from build123d import *

# Parameters (mm, degrees)
F0_W      = 125
F0_H      = 110
F1_DEPTH  = 200
F2_W      = 115.000002
F2_H      = 190.000002
F3_DEPTH  = 95
F4_R      = 2
F5_R      = 20
F7_DEPTH  = 200.001
F6_R      = 12.5
F8_DEPTH  = 200.001
F9_W      = 3
F9_H      = 190.000002
F10_DEPTH = 95


with BuildPart() as f1:
    # F0 (on Front) → F1 (new body)
    with BuildSketch(Plane.XZ):
        with Locations((62.5, 55)):
            Rectangle(F0_W, F0_H)
    extrude(amount=F1_DEPTH)

    # F2 (on face) → F3 (cut)
    with BuildSketch(Plane.XY.offset(110)):
        with Locations((62.500001, -100.000001)):
            Rectangle(F2_W, F2_H)
    extrude(amount=-F3_DEPTH, mode=Mode.SUBTRACT)

    # F4
    f4_edges = [f1.edges().sort_by_distance(p)[0] for p in [
        (125, 0, 55),
        (0, 0, 55),
        (125, -200, 55),
        (0, -200, 55),
    ]]
    fillet(f4_edges, radius=F4_R)

    # F5 (on face) → F7 (cut, through all)
    with BuildSketch(Plane.XZ.offset(200)):
        with Locations((76.975974, 50)):
            Circle(F5_R)
    extrude(amount=-F7_DEPTH, mode=Mode.SUBTRACT)

    # F6 (on face) → F8 (cut, through all)
    with BuildSketch(Plane.XZ.offset(200)):
        with Locations((22.27135, 48.594251)):
            Circle(F6_R)
        with Locations((33.396717, 82.181148)):
            Circle(F6_R)
    extrude(amount=-F8_DEPTH, mode=Mode.SUBTRACT)

    # F9 (on face) → F10 (cut, through all)
    with BuildSketch(Plane.XY.offset(110)):
        with Locations((3.5, -100.000001)):
            Rectangle(F9_W, F9_H)
    extrude(amount=-F10_DEPTH, mode=Mode.SUBTRACT)


solid = f1.part
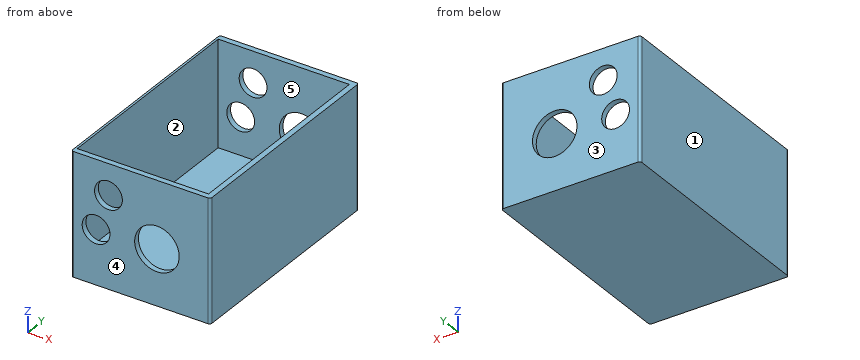
Model file for the job. Use its own axes, mm. Face numbers are marked on the shaded views. A direction names the side the tool comes from. Give positions to 0.01 mm unless a question says otherwise; leave off trailing zeros. Order: outer loops, then holes, each group sorted by start corner. A loop starts at its lowest first (then second) coordinate and runs counter-clockwise, first axis right, second up. Notation, with made-up numbers: (6.5, -21.75) - (64.5, -21.75) arc R21 ccw to (64.5, 9.25) - close; hole circle Ø2 at (77, 86). An arc over 180 degrees is marked (long way). Return JSON: item names as keys, results as strings.
1) Cut at D-D, the plane x = 32. Give the cut face in (y, z), plus the area to 3 significant figures.
Geometry says:
{"outline": "(-200, 0) - (0, 0) - (0, 40.75) - (-5, 40.75) - (-5, 15) - (-195, 15) - (-195, 40.75) - (-200, 40.75) - close; (-200, 56.44) - (-195, 56.44) - (-195, 69.76) - (-200, 69.76) - close; (-200, 94.6) - (-195, 94.6) - (-195, 110) - (-200, 110) - close; (-5, 56.44) - (0, 56.44) - (0, 69.76) - (-5, 69.76) - close; (-5, 94.6) - (0, 94.6) - (0, 110) - (-5, 110) - close", "area": "3,540 mm²"}
2) Flat gauge pins, fed straight in: P1, Ø20, axis at x = 22.27, z = 48.59, coming from the -Y side; P2, Ø2, axis at x = 64, y = -167, coming from the +Z side. Where does each tip first touch, or does it go through?
Geometry says:
{"P1": "through", "P2": "z = 15"}
3) Cut at A-A, the plane x = 66. Give the cut face in (y, z), plus the area to 3 significant figures.
Geometry says:
{"outline": "(-200, 0) - (0, 0) - (0, 33.28) - (-5, 33.28) - (-5, 15) - (-195, 15) - (-195, 33.28) - (-200, 33.28) - close; (-200, 66.72) - (-195, 66.72) - (-195, 110) - (-200, 110) - close; (-5, 66.72) - (0, 66.72) - (0, 110) - (-5, 110) - close", "area": "3,620 mm²"}
4) Cut at C-C, the plane z = 44.5. Give the cut face in (x, y), plus the area to 3 significant figures.
Geometry says:
{"outline": "(0, -198) arc R2 ccw to (2, -200) - (10.46, -200) - (10.46, -195) - (2, -195) - (2, -5) - (10.46, -5) - (10.46, 0) - (2, 0) arc R2 ccw to (0, -2) - close; (34.08, -200) - (57.75, -200) - (57.75, -195) - (34.08, -195) - close; (34.08, -5) - (57.75, -5) - (57.75, 0) - (34.08, 0) - close; (96.2, -200) - (123, -200) arc R2 ccw to (125, -198) - (125, -2) arc R2 ccw to (123, 0) - (96.2, 0) - (96.2, -5) - (120, -5) - (120, -195) - (96.2, -195) - close", "area": "1,960 mm²"}
5) Cut at B-B, the plane y = -27. Give the cut face in (x, z).
Geometry says:
{"outline": "(0, 0) - (125, 0) - (125, 110) - (120, 110) - (120, 15) - (2, 15) - (2, 110) - (0, 110) - close"}
6) Pull direction X, two halves, no side cores. Call the marked faces 1, 2 and 3: pulls with the +X half, pulls with the -X half, needs draft (parallel to the pull), parting line crosses it, or undercut.
Geometry says:
{"face 1": "pulls with the -X half", "face 2": "undercut", "face 3": "needs draft"}
7) 3-axis set-ups, long thin cutter, end or side, ignore diameter. For the marked faces 4 and 5: which of +Z, -Z, +X, -X, +Y, -Y reach the whole face in a straight line?
Geometry says:
{"face 4": "+Z, -Z, +X, -X, -Y", "face 5": "+Z"}
8) Probe line 1 (Y direction, x = 118, z = 58.5); line 2 (X direction, y = -16, z = 87.5); line 3 (Z direction, x = 103, y = -58). List the from-to ranges inside material, lowest first. Write a range as from..to.
Geometry says:
{"line 1": "-200..-195, -5..0", "line 2": "0..2, 120..125", "line 3": "0..15"}
